Could you check a few things on this model? Use its own coordinates, in mm. A direction names the side the tool comes from. Coordinates: 2 decimals unless noted, no trailing zeros. Loops run counter-clockwise (first coordinate to the right, second up) from the corner with the lowest first, then second, coordinate; pieces in that order, holes last. Notation, with made-up numbers: (-14.5, -1) - (-5.5, -1) arc R30 cw to (-5.5, 25) - close; hole circle Ø6 at (4.5, 65.25). An arc over 180 degrees is marked (long way). One line per item, written item: value. Start each with the question number.
(1) If I drill on line 1 along Z through (x, y) = (-78, 16); line 2 along Z through (x, y) = (-146.5, 6.5); line 3 along Y through (x, z) = (-158, 100), over which ranges is the centre line in solid material (lowest first)? Write a range as from..to.
(2) I'm going to push flat-ended pins straight in: P1, Ø4.5, axis at x = -119.5, z = 82.5, coming from the -Y side; P2, Ø3, axis at x = -125, y = 14.5, coming from the -Z side; P3, Ø10, axis at x = -115.5, z = 119.5, coming from the +Y side; P4, Ø6.5, axis at y = 5, z = 186.5, coming from the +X side (3 decimals). Where does each tip first touch, or does it pass through?
(3) If we section it at C-C on y = 4: Write out the boundary of the cut face in (x, z) (3 decimals).
(4) If we mould it in two halves opening along X, with no side actions, what happens to faces 1 (the face through (-161.925, 7, 184)), 2 (the face through (-98.425, 9, 6)), 3 (the face through (-123, 6.35, 89))? For each: pulls with the +X half, pulls with the -X half, needs draft (parallel to the pull), parting line crosses it, or undercut.
(5) If we section it at B-B on x = -148: Write out the boundary of the cut face in (y, z), then the cut area to 3 significant figures.
(6) If we section it at D-D on z = 119: Write out the boundary of the cut face in (x, y) (3 decimals).
(7) On a 3-axis mill with a long thin cutter (end or side, diameter ignored), from which of +Z, -Z, +X, -X, +Y, -Y can I reach the whole of each face in a straight line? I mean faces 4 (the face through (-102, 9, 12.7)), 5 (the face through (-123, 16, 114.3)), 6 (the face through (-123, 10, 80.162)), 7 (the face through (-89, 10, 177.8)). Say none if no direction works.
(8) If we section it at A-A on y = 15: Write out the boundary of the cut face in (x, z) (1 decimal), then the cut area to 3 significant figures.
Autodesk Inventor part; units mm, degrees
ref_plane "YZ Plane" through (0, 0, 0) normal (1, 0, 0) x (0, 1, 0)
ref_plane "XZ Plane" through (0, 0, 0) normal (0, 1, 0) x (-1, 0, 0)
sketch "Sketch3" plane through (0, 0, 0) normal (0, 0, 1) x (1, 0, 0)
  line L0 (0, -9.525) -> (9.525, -9.525)
  line L1 (9.525, -9.525) -> (9.525, 0)
  line L2 (0, 0) -> (0, -9.525) construction
  line L3 (0, 0) -> (9.525, 0) construction
  line L4 (0, -9.525) -> (-9.525, -9.525)
  line L5 (-9.525, -9.525) -> (-9.525, 0)
  line L6 (9.525, 0) -> (73.025, 0)
  line L7 (-187.325, 0) -> (-187.325, 19.05)
  line L8 (-187.325, 0) -> (-9.525, 0)
  line L9 (73.025, 0) -> (73.025, 19.05)
  line L10 (73.025, 19.05) -> (-187.325, 19.05)
  dimension "d0" = 9.525
  dimension "d1" = 9.525
  dimension "d6" = 63.5
  dimension "d8" = 19.05
  dimension "d9" = 177.8
extrude "Extrusion1" add sketch "Sketch3" along normal mid plane 355.6
sketch "Sketch4" plane through (0, 0, 177.8) normal (0, 0, 1) x (1, 0, 0)
  line L0 (-187.325, 19.05) -> (73.025, 19.05) construction
  line L1 (0, 19.05) -> (0, -9.525) construction
  line L2 (9.525, -9.525) -> (-9.525, -9.525) construction
  line L3 (0, -9.525) -> (-22.225, -9.525)
  line L4 (-22.225, -9.525) -> (-22.225, 19.05)
  line L5 (-22.225, 19.05) -> (0, 19.05)
  line L6 (187.325, 19.05) -> (-73.025, 19.05) construction
  line L7 (0, -9.525) -> (22.225, -9.525)
  line L8 (22.225, -9.525) -> (22.225, 19.05)
  line L9 (0, 19.05) -> (22.225, 19.05)
  point P0 (0, 0)
  dimension "d12" = 22.225
extrude "Extrusion2" add sketch "Sketch4" along normal blind 12.7
mirror "Mirror1" about plane through (0, 0, 0) normal (0, 0, 1) of "Extrusion2"
sketch "Sketch6" plane through (-187.325, 0, -177.8) normal (0, -1, 0) x (1, 0, 0)
  line L0 (82.55, 165.1) -> (88.9, 165.1)
  line L1 (88.9, 165.1) -> (88.9, 190.5)
  line L2 (88.9, 190.5) -> (82.55, 190.5)
  line L3 (82.55, 190.5) -> (82.55, 165.1)
  line L4 (82.55, 165.1) -> (88.9, 190.5) construction
  line L5 (88.9, 165.1) -> (82.55, 190.5) construction
  line L6 (177.8, 0) -> (177.8, 355.6)
  point P0 (187.325, 177.8)
  point P1 (85.725, 177.8)
  dimension "d16" = 12.7
  dimension "d18" = 6.35
  dimension "d19" = 88.9
extrude "Extrusion3" cut sketch "Sketch6" against normal through all
sketch "Sketch7" plane through (0, 0, 177.8) normal (0, 0, 1) x (1, 0, 0)
  line L0 (-187.325, 19.05) -> (-22.225, 19.05)
  line L1 (-161.925, 19.05) -> (-117.475, 19.05)
  line L2 (-117.475, 19.05) -> (-117.475, -3.81)
  line L3 (-117.475, -3.81) -> (-161.925, -3.81)
  line L4 (-161.925, -3.81) -> (-161.925, 19.05)
  line L5 (-187.325, 19.05) -> (-187.325, 0)
  point P0 (0, 0)
  dimension "d22" = 44.45
  dimension "d23" = 22.86
  dimension "d24" = 25.4
extrude "Extrusion4" add sketch "Sketch7" along normal blind 12.7
mirror "Mirror2" about plane through (0, 0, 0) normal (0, 0, 1) of "Extrusion4"
sketch "Sketch9" plane through (73.025, 0, 177.8) normal (1, 0, 0) x (0, 0, -1)
  line L0 (355.6, 19.05) -> (0, 19.05)
  line L1 (50.8, 19.05) -> (63.5, 19.05)
  line L2 (63.5, 19.05) -> (63.5, 12.7)
  line L3 (63.5, 12.7) -> (50.8, 12.7)
  line L4 (50.8, 12.7) -> (50.8, 19.05)
  line L5 (0, 0) -> (0, 19.05)
  point P0 (177.8, 0)
  dimension "d28" = 12.7
  dimension "d29" = 6.35
  dimension "d30" = 50.8
extrude "Extrusion5" cut sketch "Sketch9" against normal through all
mirror "Mirror3" about plane through (0, 0, 0) normal (0, 0, 1) of "Extrusion5"
sketch "Sketch12" plane through (73.025, 0, 177.8) normal (1, 0, 0) x (0, 0, -1)
  line L0 (355.6, 0) -> (0, 0) construction
  line L1 (88.9, 0) -> (88.9, 16.5009) construction
  line L2 (0, 0) -> (0, 19.05)
  line L3 (50.8, 19.05) -> (0, 19.05)
  line L4 (84.1375, 19.05) -> (84.1375, 12.7)
  line L5 (84.1375, 12.7) -> (80.1624, 12.7)
  line L6 (80.1624, 12.7) -> (80.1624, 6.35)
  line L7 (80.1624, 6.35) -> (88.9, 6.35)
  line L8 (93.6625, 19.05) -> (93.6625, 12.7)
  line L9 (93.6625, 12.7) -> (97.6376, 12.7)
  line L10 (97.6376, 12.7) -> (97.6376, 6.35)
  line L11 (97.6376, 6.35) -> (88.9, 6.35)
  line L12 (84.1375, 19.05) -> (93.6625, 19.05)
  point P0 (177.8, 0)
  dimension "d46" = 88.9
  dimension "d47" = 4.7625
  dimension "d48" = 6.35
  dimension "d49" = 6.35
  dimension "d50" = 8.7376
extrude "Extrusion8" cut sketch "Sketch12" against normal through all
mirror "Mirror4" about plane through (0, 0, 0) normal (0, 0, 1) of "Extrusion8"
split "Split2" plane through (0, 0, 0) removes the side toward (0, 0, -1)
ref_plane "Work Plane1" through (-60.325, 0, 177.8) normal (1, 0, 0) x (0, 0, -1)
split "Split3" plane through (-60.325, 0, 177.8) removes the side toward (1, 0, 0)
properties part number "BandSawJigBottomSpiltA-SplitB" material "LCP Plastic"
Values:
1. line 1: z = 0..84.14, 93.66..114.3, 127..177.8
1. line 2: z = 0..80.16, 97.64..190.5
1. line 3: y = 0..19.05
2. P1: stops at y = 0
2. P2: stops at z = 0
2. P3: stops at y = 12.7
2. P4: stops at x = -117.475
3. outline: (-187.325, 0) - (-104.775, 0) - (-104.775, 12.7) - (-98.425, 12.7) - (-98.425, 0) - (-60.325, 0) - (-60.325, 177.8) - (-117.475, 177.8) - (-117.475, 190.5) - (-161.925, 190.5) - (-161.925, 177.8) - (-187.325, 177.8) - close
4. face 1: pulls with the -X half
4. face 2: undercut
4. face 3: needs draft
5. outline: (-3.81, 177.8) - (0, 177.8) - (0, 0) - (19.05, 0) - (19.05, 84.14) - (12.7, 84.14) - (12.7, 80.16) - (6.35, 80.16) - (6.35, 97.64) - (12.7, 97.64) - (12.7, 93.66) - (19.05, 93.66) - (19.05, 114.3) - (12.7, 114.3) - (12.7, 127) - (19.05, 127) - (19.05, 190.5) - (-3.81, 190.5) - close
5. area: 3,430 mm2
6. outline: (-187.325, 0) - (-60.325, 0) - (-60.325, 12.7) - (-187.325, 12.7) - close
7. face 4: -Z, +Y, -Y
7. face 5: +X, -X, +Y
7. face 6: +X, -X
7. face 7: +Z, +X, +Y, -Y
8. outline: (-187.3, 0) - (-104.8, 0) - (-104.8, 12.7) - (-98.4, 12.7) - (-98.4, 0) - (-60.3, 0) - (-60.3, 84.1) - (-187.3, 84.1) - close; (-187.3, 93.7) - (-60.3, 93.7) - (-60.3, 114.3) - (-187.3, 114.3) - close; (-187.3, 127) - (-60.3, 127) - (-60.3, 177.8) - (-117.5, 177.8) - (-117.5, 190.5) - (-161.9, 190.5) - (-161.9, 177.8) - (-187.3, 177.8) - close
8. area: 20,200 mm2
